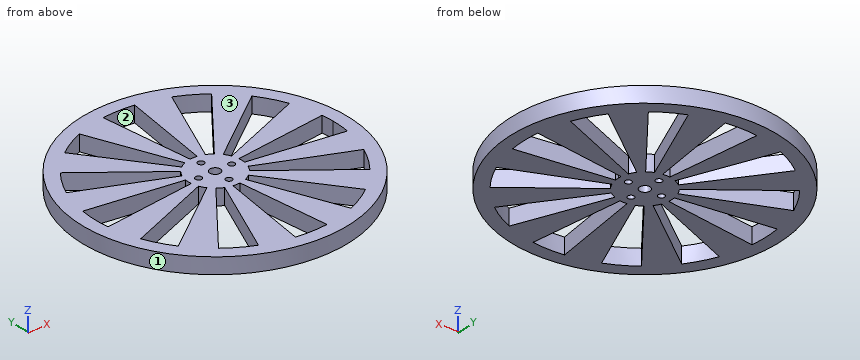
from build123d import *

# Parameters (mm, degrees)
SKETCH2_R           = 63.5
BOSS_EXTRUDE1_DEPTH = 7.62
CUT_EXTRUDE3_DEPTH  = 91.125270596
SKETCH6_R           = 1.5
CUT_EXTRUDE6_DEPTH  = 91.125270596
CIRPATTERN1_COUNT   = 4
SKETCH7_R           = 2.5
CUT_EXTRUDE5_DEPTH  = 91.125270596


with BuildPart() as part:
    # Sketch2 → Boss-Extrude1 (new body)
    with BuildSketch(Plane.XY):
        with Locations(Location((0, 0, 0), (0, 0, 180))):
            Circle(SKETCH2_R)
    extrude(amount=BOSS_EXTRUDE1_DEPTH)

    # Sketch5 → Cut-Extrude3 (cut, through all)
    with BuildSketch(Plane.XY.offset(7.62)):
        with BuildLine():
            ThreePointArc((-1.318093472, 12.631414394), (0.341913424, 12.695396615), (1.996070086, 12.54215708))
            Line((1.996070086, 12.54215708), (8.982315386, 56.439706859))
            ThreePointArc((8.982315386, 56.439706859), (1.538610407, 57.129284767), (-5.931420623, 56.841364774))
            Line((-5.931420623, 56.841364774), (-1.318093472, 12.631414394))
        make_face()
        with BuildLine():
            Line((23.283921447, 52.191776192), (5.174204766, 11.598172487))
            ThreePointArc((5.174204766, 11.598172487), (6.643804018, 10.823579268), (7.999725942, 9.863791606))
            Line((7.999725942, 9.863791606), (35.998766739, 44.387062229))
            ThreePointArc((35.998766739, 44.387062229), (29.897118082, 48.706106705), (23.283921447, 52.191776192))
        make_face()
        with BuildLine():
            ThreePointArc((10.280079015, 7.457209628), (11.165492692, 6.051592597), (11.859861692, 4.542431138))
            Line((11.859861692, 4.542431138), (53.369377615, 20.44094012))
            ThreePointArc((53.369377615, 20.44094012), (50.244717112, 27.232166685), (46.260355568, 33.557443327))
            Line((46.260355568, 33.557443327), (10.280079015, 7.457209628))
        make_face()
        with BuildLine():
            ThreePointArc((12.7, 0), (12.660477774, -1.00115061), (12.54215708, -1.996070086))
            Line((12.54215708, -1.996070086), (56.439706859, -8.982315386))
            ThreePointArc((56.439706859, -8.982315386), (56.972149981, -4.505177745), (57.15, 0))
            ThreePointArc((57.15, 0), (57.072789037, 2.969722475), (56.841364774, 5.931420623))
            Line((56.841364774, 5.931420623), (12.631414394, 1.318093472))
            ThreePointArc((12.631414394, 1.318093472), (12.682842008, 0.659938328), (12.7, 0))
        make_face()
        with BuildLine():
            ThreePointArc((11.598172487, -5.174204766), (10.823579268, -6.643804018), (9.863791606, -7.999725942))
            Line((9.863791606, -7.999725942), (44.387062229, -35.998766739))
            ThreePointArc((44.387062229, -35.998766739), (48.706106705, -29.897118082), (52.191776192, -23.283921447))
            Line((52.191776192, -23.283921447), (11.598172487, -5.174204766))
        make_face()
        with BuildLine():
            ThreePointArc((7.457209628, -10.280079015), (6.051592597, -11.165492692), (4.542431138, -11.859861692))
            Line((4.542431138, -11.859861692), (20.44094012, -53.369377615))
            ThreePointArc((20.44094012, -53.369377615), (27.232166685, -50.244717112), (33.557443327, -46.260355568))
            Line((33.557443327, -46.260355568), (7.457209628, -10.280079015))
        make_face()
        with BuildLine():
            ThreePointArc((1.318093472, -12.631414394), (-0.341913424, -12.695396615), (-1.996070086, -12.54215708))
            Line((-1.996070086, -12.54215708), (-8.982315386, -56.439706859))
            ThreePointArc((-8.982315386, -56.439706859), (-1.538610407, -57.129284767), (5.931420623, -56.841364774))
            Line((5.931420623, -56.841364774), (1.318093472, -12.631414394))
        make_face()
        with BuildLine():
            ThreePointArc((-5.174204766, -11.598172487), (-6.643804018, -10.823579268), (-7.999725942, -9.863791606))
            Line((-7.999725942, -9.863791606), (-35.998766739, -44.387062229))
            ThreePointArc((-35.998766739, -44.387062229), (-29.897118082, -48.706106705), (-23.283921447, -52.191776192))
            Line((-23.283921447, -52.191776192), (-5.174204766, -11.598172487))
        make_face()
        with BuildLine():
            ThreePointArc((-10.280079015, -7.457209628), (-11.165492692, -6.051592597), (-11.859861692, -4.542431138))
            Line((-11.859861692, -4.542431138), (-53.369377615, -20.44094012))
            ThreePointArc((-53.369377615, -20.44094012), (-50.244717112, -27.232166685), (-46.260355568, -33.557443327))
            Line((-46.260355568, -33.557443327), (-10.280079015, -7.457209628))
        make_face()
        with BuildLine():
            ThreePointArc((-12.631414394, -1.318093472), (-12.695396615, 0.341913424), (-12.54215708, 1.996070086))
            Line((-12.54215708, 1.996070086), (-56.439706859, 8.982315386))
            ThreePointArc((-56.439706859, 8.982315386), (-57.129284767, 1.538610407), (-56.841364774, -5.931420623))
            Line((-56.841364774, -5.931420623), (-12.631414394, -1.318093472))
        make_face()
        with BuildLine():
            ThreePointArc((-11.598172487, 5.174204766), (-10.823579268, 6.643804018), (-9.863791606, 7.999725942))
            Line((-9.863791606, 7.999725942), (-44.387062229, 35.998766739))
            ThreePointArc((-44.387062229, 35.998766739), (-48.706106705, 29.897118082), (-52.191776192, 23.283921447))
            Line((-52.191776192, 23.283921447), (-11.598172487, 5.174204766))
        make_face()
        with BuildLine():
            ThreePointArc((-7.457209628, 10.280079015), (-6.051592597, 11.165492692), (-4.542431138, 11.859861692))
            Line((-4.542431138, 11.859861692), (-20.44094012, 53.369377615))
            ThreePointArc((-20.44094012, 53.369377615), (-27.232166685, 50.244717112), (-33.557443327, 46.260355568))
            Line((-33.557443327, 46.260355568), (-7.457209628, 10.280079015))
        make_face()
    extrude(amount=-CUT_EXTRUDE3_DEPTH, mode=Mode.SUBTRACT)

    # Sketch6 → Cut-Extrude6 (cut, through all)
    with BuildSketch(Plane.XY.offset(7.62)):
        with Locations((0, 8)):
            Circle(SKETCH6_R)
    cut_extrude6 = extrude(amount=-CUT_EXTRUDE6_DEPTH, mode=Mode.SUBTRACT)

    # CirPattern1: Cut-Extrude6 ×4 about axis
    cirpattern1_axis = Axis((0, 0, 0), (0, 0, 1))
    for i in range(1, CIRPATTERN1_COUNT):
        add(cut_extrude6.rotate(cirpattern1_axis, i * 360 / CIRPATTERN1_COUNT), mode=Mode.SUBTRACT)

    # Sketch7 → Cut-Extrude5 (cut, through all)
    with BuildSketch(Plane.XY.offset(7.62)):
        Circle(SKETCH7_R)
    extrude(amount=-CUT_EXTRUDE5_DEPTH, mode=Mode.SUBTRACT)


solid = part.part
Can you work these out from the model? Positions are in its coordinate system, mm. Face numbers are marked on the shaded views. Coordinates: 2 decimals unless noted, no trailing zeros. Loops run counter-clockwise (first coordinate to the right, second up) from the corner with the lowest first, then second, coordinate; pieces in that order, holes last. Notation, with made-up numbers: (15.5, -38) - (42.5, -38) arc R5 ccw to (42.5, -33) - close; hole circle Ø10 at (84, 60.25). An arc over 180 degrees is marked (long way). Answer as a JSON object with one key per item and string values. Group by question number.
Item 1: If we mould it in two halves opening along X, with no side actions, what happens to the marked faces 1, 2 and 3? For each: released by +X, released by -X, zero draft, split by the parting line, or undercut.
Item 2: For pin 1 (3 mm diameter, centred on x = 12, z = 1.5, fed in from -Y); pin 2 (4 mm diameter, centred on x = 7, z = 5, fed in from +Y); pin 3 (3 mm diameter, centred on y = -29, z = 3, fed in from -X), each with a flat end and sliding along its axis, tell me the tip position at first contact or that it passes through.
Item 3: If we section it at B-B (x = -15): List the corners of the cut face in (y, z) for me.
Item 4: If I drill on L1, parallel to Y at x = 0, z = 2.75; L2, parallel to X at y = 47, z = 4; L3, parallel to X at y = -43, z = 4.25, over which ranges is the centre line in solid material (lowest first)? Write a range as from..to.
Item 5: If we section it at A-A (y = -29.5): List the corners of the cut face in (x, z) for me.
Item 6: If we section it at C-C (z = 4): State how many separate pieces and enclosed holes the cut face has, plus the area to 3 significant figures.
Returned:
{
 "1": {"face 1": "split by the parting line", "face 2": "undercut", "face 3": "zero draft"},
 "2": {"pin 1": "stops at y = -62.63", "pin 2": "stops at y = 63.3", "pin 3": "stops at x = -57.24"},
 "3": {"outline": "(-61.7, 0) - (-33.62, 0) - (-33.62, 7.62) - (-61.7, 7.62) - close; (-18.5, 0) - (-10.88, 0) - (-10.88, 7.62) - (-18.5, 7.62) - close; (-5.75, 0) - (-1.57, 0) - (-1.57, 7.62) - (-5.75, 7.62) - close; (2.39, 0) - (6.69, 0) - (6.69, 7.62) - (2.39, 7.62) - close; (12.17, 0) - (20.68, 0) - (20.68, 7.62) - (12.17, 7.62) - close; (39.16, 0) - (61.7, 0) - (61.7, 7.62) - (39.16, 7.62) - close"},
 "4": {"L1": "y = -63.5..-57.15, -12.7..-9.5, -6.5..-2.5, 2.5..6.5, 9.5..12.7, 57.15..63.5", "L2": "x = -42.7..-32.51, -18..-4.9, 7.48..20.97, 32.51..42.7", "L3": "x = -46.73..-34.87, -19.18..-6.84, 4.49..16.47, 31.19..46.73"},
 "5": {"outline": "(-56.23, 0) - (-48.95, 0) - (-48.95, 7.62) - (-56.23, 7.62) - close; (-40.67, 0) - (-23.93, 0) - (-23.93, 7.62) - (-40.67, 7.62) - close; (-13.16, 0) - (-4.69, 0) - (-4.69, 7.62) - (-13.16, 7.62) - close; (3.08, 0) - (11.3, 0) - (11.3, 7.62) - (3.08, 7.62) - close; (21.4, 0) - (36.37, 0) - (36.37, 7.62) - (21.4, 7.62) - close; (48.95, 0) - (56.23, 0) - (56.23, 7.62) - (48.95, 7.62) - close"},
 "6": {"separate pieces": "1", "enclosed holes": "17", "area": "7,740 mm²"}
}
